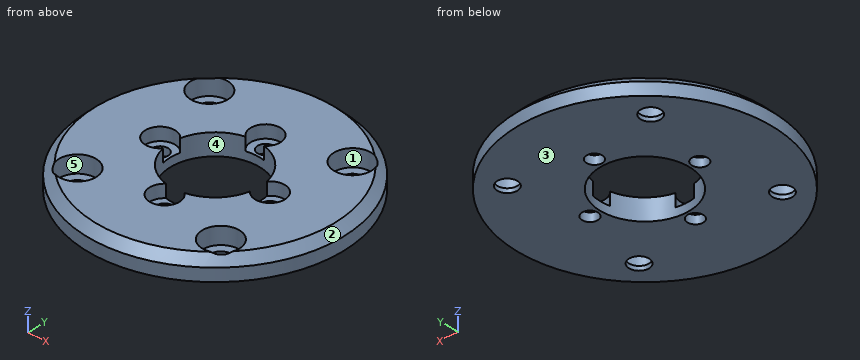
from build123d import *

# Parameters (mm, degrees)
F0_R           = 30
F0_R_2         = 10.5
F1_DEPTH       = 5
F3_D           = 4.7
F3_CBORE_D     = 8.75
F3_CBORE_DEPTH = 4
F5_D           = 3.7
F5_CBORE_D     = 7
F5_CBORE_DEPTH = 3


# Not quite as in the source:
# - a fillet or chamfer that OpenCascade refuses, or shapes differently, is made with other operations: its cross-section is extruded or revolved along the edge and cut away or added


with BuildPart() as f1:
    # F0 (on Top) → F1 (new body)
    with BuildSketch(Plane.XY):
        Circle(F0_R)
        Circle(F0_R_2, mode=Mode.SUBTRACT)
    extrude(amount=F1_DEPTH)

    # F3 (through all)
    with Locations(Plane.XY.offset(5)):
        with Locations((-16.9705627485, 16.9705627485), (16.9705627485, 16.9705627485), (16.9705627485, -16.9705627485), (-16.9705627485, -16.9705627485)):
            CounterBoreHole(F3_D / 2, F3_CBORE_D / 2, F3_CBORE_DEPTH)

    # F5 (through all)
    with Locations(Plane.XY.offset(5)):
        with Locations((0, 13), (-13, 0), (0, -13), (13, 0)):
            CounterBoreHole(F5_D / 2, F5_CBORE_D / 2, F5_CBORE_DEPTH)

    # F6: chamfer of 2 on 1 edges, made by hand

    # F6_s1 → F6_t2 (revolve, cut)
    with BuildSketch(Plane.XZ):
        Polygon((30, 3), (28, 5), (30, 5), align=None)
    revolve(axis=Axis((0, 0, 5), (0, 0, 1)), mode=Mode.SUBTRACT)


solid = f1.part
Geometry check sheet. Reference: the model listing, model coordinates, mm. Face numbers are marked on the shaded views. A direction names the side the tool comes from. Give positions to 0.01 mm unless a question says otherwise; leave off trailing zeros. Order: outer loops, then holes, each group sorted by start corner. A loop starts at its lowest first (then second) coordinate and runs counter-clockwise, first axis right, second up.
1. Scan lines: line 1 (Y direction, x = -15, z = 2.35); line 2 (X direction, y = 14, z = 1.4); line 3 (X direction, y = 1, z = 1.1). Record each from-to range of solid material in increasing order.
Completed:
line 1: y = -25.98 to -20.88, -13.06 to -2.87, 2.87 to 13.06, 20.88 to 25.98
line 2: x = -26.53 to -20.18, -13.76 to -1.56, 1.56 to 13.76, 20.18 to 26.53
line 3: x = -29.98 to -14.56, -11.44 to -10.45, 10.45 to 11.44, 14.56 to 29.98
2. Depth check by flat-ended pin: pin 1 (4 mm diameter, centred on x = 0, y = -13, fed in from +Z); pin 2 (2 mm diameter, centred on x = 0, y = -13, fed in from +Z); pin 3 (3 mm diameter, centred on y = 9, z = 4, fed in from +X); pin 4 (8 mm diameter, centred on x = -16.97, y = 16.97, fed in from +Z). Enter the tip coordinate at first touch or a pass-through.
Completed:
pin 1: stops at z = 2
pin 2: passes through
pin 3: stops at x = 28.95
pin 4: stops at z = 1
3. Draft check along X on the marked faces 1, 2 and 3. Enter one of: pulls with the +X half, pulls with the -X half, needs draft (parallel to the pull), parting line crosses it, or undercut.
Completed:
face 1: undercut
face 2: parting line crosses it
face 3: needs draft
4. Access from +Z, -Z, +X, -X, +Y, -Y to the whole of each face (thin tool, end or side, straight path). Record for the marked faces 4 and 5.
Completed:
face 4: +Z, -Z
face 5: +Z
5. Sectioned sample at A-A (y = 0). Record the boundary of the cut face in (x, z), then the cut area to 3 significant figures.
Completed:
outline: (-30, 0) - (-14.85, 0) - (-14.85, 2) - (-16.5, 2) - (-16.5, 5) - (-28, 5) - (-30, 3) - close; (-11.15, 0) - (-10.5, 0) - (-10.5, 2) - (-11.15, 2) - close; (10.5, 0) - (11.15, 0) - (11.15, 2) - (10.5, 2) - close; (14.85, 0) - (30, 0) - (30, 3) - (28, 5) - (16.5, 5) - (16.5, 2) - (14.85, 2) - close
area: 140 mm2
